```python
from build123d import *

# Parameters (mm, degrees)
F0_R          = 4.7625
F0_R_2        = 3.175
F1_DEPTH      = 3.175
F2_R          = 12.7
F3_DEPTH      = 31.75
F3_DEPTH_BACK = 28.575


with BuildPart() as f1:
    # F0 (on Right) → F1 (new body)
    with BuildSketch(Plane.YZ):
        with BuildLine():
            Line((194.222937, -75.896066), (199.837454, -52.714848))
            ThreePointArc((199.837454, -52.714848), (197.343361, -50.871673), (197.273806, -47.771197))
            ThreePointArc((197.273806, -47.771197), (192.906665, -47.242193), (188.611001, -48.190366))
            ThreePointArc((188.611001, -48.190366), (127.959227, -56.863753), (66.740255, -59.334101))
            ThreePointArc((66.740255, -59.334101), (43.22785, -56.518652), (58.68969, -74.45441))
            ThreePointArc((58.68969, -74.45441), (118.843076, -65.773207), (179.537445, -68.93336))
            ThreePointArc((179.537445, -68.93336), (187.206277, -71.726944), (194.222937, -75.896066))
        make_face()
        with Locations((54.437917, -62.487271)):
            Circle(F0_R, mode=Mode.SUBTRACT)
        Polygon((265.879052, -64.764367), (199.837454, -52.714848), (194.222937, -75.896066), (265.879052, -88.969973), align=None)
        with Locations((259.567566, -75.763282)):
            Circle(F0_R_2, mode=Mode.SUBTRACT)
        with Locations((216.053504, -66.689754)):
            Circle(F0_R_2, mode=Mode.SUBTRACT)
    extrude(amount=F1_DEPTH)

    # F2 (on Right) → F3 (join, two sides)
    with BuildSketch(Plane.YZ) as f3_sk:
        with Locations((54.437917, -62.487271)):
            Circle(F2_R)
    extrude(amount=F3_DEPTH)
    extrude(f3_sk.sketch, amount=-F3_DEPTH_BACK)


solid = f1.part
```
Model file for the job. Use its own axes, mm. A direction names the side the tool comes from. Give positions to 0.01 mm unless a question says otherwise; leave off trailing zeros. Loops run counter-clockwise (first coordinate to the right, second up) from the corner with the lowest first, then second, coordinate; pieces in that order, holes last. Notation, with made-up numbers: (29.25, -18) - (73.25, -18) arc R18 cw to (73.25, 17) - close; hole circle Ø10 at (69.25, -20.5). An arc over 180 degrees is marked (long way). One line per item, written item: value. Start each with the question number.
1. Slice it at C-C (x = 12.5). List the corners of the cut face in (y, z).
2. Pin check, flat tips, straight feed: pin 1 (1.5 mm diameter, centred on x = 2, z = -71.5, fed in from -Y); pin 2 (12.5 mm diameter, centred on y = 118, z = -73.5, fed in from +X); pin 3 (8.5 mm diameter, centred on y = 216.05, z = -66.69, fed in from +X) (3 decimals); pin 4 (4 mm diameter, centred on x = 19, z = -60, fed in from +Y). Stop position of each tip, or through.
3. Slice it at B-B (y = 147). List the corners of the cut face in (x, z) (3 decimals).
4. Pull direction Z, two halves, no side cores. Call faces 1 (the cylindrical face through (1.565, 219.082, -65.736)), 2 (the cylindrical face through (1.565, 117.992, -65.813)), 3 (the flat face through (-28.575, 54, -62)), 4 (the flat face through (1.565, 233.321, -58.824)): pulls with the +Z half, pulls with the -Z half, needs draft (parallel to the pull), parting line crosses it, or undercut.
5. Slice it at A-A (y = 216). List the corners of the cut face in (x, z) (3 decimals), plus the area to 3 significant figures.
6. Probe L1, parallel to X at y = 251.5, z = -71 (3 decimals); L2, parallel to Z at x = -13, y = 58; L3, parallel to Y at x = -0.5, z = -53. List the from-to ranges inside material, lowest first. Write a range as from..to.
7. Slice it at D-D (y = 95.5). List the corners of the cut face in (x, z) (3 decimals).
8. Which spindle directions (+Z, -Z, +X, -X, +Y, -Y) get a long thin tool onto all of the face, cutting with end or side? Do faces 5 (the cylindrical face through (1.565, 128.814, -56.785)), 6 (the flat face through (1.57, 229.55, -82.34)), 7 (the cylindrical face through (1.565, 187.103, -71.678)). Say none if no direction does.
Solution:
1. outline: circle Ø25.4 at (54.44, -62.49)
2. pin 1: stops at y = 44.79
2. pin 2: passes through
2. pin 3: stops at x = 3.175
2. pin 4: stops at y = 67.13
3. outline: (0, -65.76) - (3.175, -65.76) - (3.175, -54.817) - (0, -54.817) - close
4. face 1: undercut
4. face 2: pulls with the -Z half
4. face 3: needs draft
4. face 4: pulls with the +Z half
5. outline: (0, -79.869) - (3.175, -79.869) - (3.175, -69.864) - (0, -69.864) - close; (0, -63.515) - (3.175, -63.515) - (3.175, -55.664) - (0, -55.664) - close
5. area: 56.7 mm^2
6. L1: x = 0..3.175
6. L2: z = -74.68..-50.3
6. L3: y = 46..62.88
7. outline: (0, -67.721) - (3.175, -67.721) - (3.175, -58.95) - (0, -58.95) - close
8. face 5: +Z, +X, -X
8. face 6: -Z, +X, -X, -Y
8. face 7: -Z, +X, -X
